from build123d import *

# Parameters (mm, degrees)
CROQUIS1_R               = 0.5
SALIENTE_EXTRUIR1_DEPTH  = 3
SALIENTE_EXTRUIR2_DEPTH  = 11
SALIENTE_EXTRUIR3_DEPTH  = 5.75
CROQUIS4_R               = 2
CROQUIS4_R_2             = 1
CORTAR_EXTRUIR1_DEPTH    = 4
SALIENTE_EXTRUIR5_START  = 4
CROQUIS6_R               = 2
CROQUIS6_R_2             = 1
SALIENTE_EXTRUIR5_DEPTH  = 4
SALIENTE_EXTRUIR6_DEPTH  = 1.5
CROQUIS9_W               = 44.5
CROQUIS9_H               = 15.5
SALIENTE_EXTRUIR7_DEPTH  = 1
CROQUIS11_W              = 10.5
CROQUIS11_H              = 15.5
SALIENTE_EXTRUIR10_DEPTH = 2
CROQUIS7_R               = 2.25
CORTAR_EXTRUIR2_DEPTH    = 2


with BuildPart() as part:
    # Croquis1 → Saliente-Extruir1 (new body)
    with BuildSketch(Plane(origin=(0, 0, 0), x_dir=(1, 0, 0), z_dir=(0, 1, 0))):
        Polygon((-6, -0.75), (-6, -5.5), (4, -5.5), (13.5, -5.5), (13.5, 26.5), (13.5, 39), (4, 39), (4, 26.5), (-6, 26.5), (-6, 21.75), (4, 21.75), (6, 21.75), (6, 11.25), (6, -0.75), align=None)
        with Locations(Location((0, -3.125, 0), (0, 0, 270))):
            Circle(CROQUIS1_R, mode=Mode.SUBTRACT)
        with Locations(Location((0, 24.125, 0), (0, 0, 270))):
            Circle(CROQUIS1_R, mode=Mode.SUBTRACT)
    extrude(amount=SALIENTE_EXTRUIR1_DEPTH)

    # Croquis2 → Saliente-Extruir2 (add)
    with BuildSketch(Plane(origin=(0, 3, 0), x_dir=(1, 0, 0), z_dir=(0, 1, 0))):
        Polygon((11.25, -5.5), (13.5, -5.5), (13.5, 26.5), (13.5, 39), (4, 39), (4, 26.5), (4, 21.75), (6, 21.75), (6, 12.75), (7.25, 12.75), (7.25, 33), (11.25, 33), align=None)
    extrude(amount=SALIENTE_EXTRUIR2_DEPTH)

    # Croquis3 → Saliente-Extruir3 (add)
    with BuildSketch(Plane(origin=(0, 3, 0), x_dir=(1, 0, 0), z_dir=(0, 1, 0))):
        Polygon((11.25, -5.5), (11.25, 33), (7.25, 33), (7.25, 12.75), (6, 12.75), (6, -5.5), align=None)
    extrude(amount=SALIENTE_EXTRUIR3_DEPTH)

    # Croquis4 → Cortar-Extruir1 (cut)
    with BuildSketch(Plane(origin=(0, 0, -39), x_dir=(-1, 0, 0), z_dir=(0, 0, -1))):
        with Locations((-9.87, 11.055)):
            Circle(CROQUIS4_R)
        with Locations((-9.87, 5.555)):
            Circle(CROQUIS4_R_2)
        with Locations((-9.87, 2.055)):
            Circle(CROQUIS4_R_2)
    extrude(amount=-CORTAR_EXTRUIR1_DEPTH, mode=Mode.SUBTRACT)

    # Croquis6 → Saliente-Extruir5 (add)
    with BuildSketch(Plane(origin=(0, 0, -35), x_dir=(-1, 0, 0), z_dir=(0, 0, -1)).offset(SALIENTE_EXTRUIR5_START)):
        with Locations((-9.87, 11.055)):
            Circle(CROQUIS6_R)
        with Locations((-9.87, 5.555)):
            Circle(CROQUIS6_R_2)
        with Locations((-9.87, 2.055)):
            Circle(CROQUIS6_R_2)
    extrude(amount=-SALIENTE_EXTRUIR5_DEPTH)

    # Croquis8 → Saliente-Extruir6 (add)
    with BuildSketch(Plane(origin=(0, 14, 0), x_dir=(1, 0, 0), z_dir=(0, 1, 0))):
        Polygon((4, 39), (4, 21.75), (6, 21.75), (6, 12.75), (7.25, 12.75), (7.25, 33), (11.25, 33), (11.25, -5.5), (13.5, -5.5), (13.5, 39), align=None)
    extrude(amount=SALIENTE_EXTRUIR6_DEPTH)

    # Croquis9 → Saliente-Extruir7 (add)
    with BuildSketch(Plane(origin=(13.5, 0, 0), x_dir=(0, 0, -1), z_dir=(1, 0, 0))):
        with Locations((16.75, 7.75)):
            Rectangle(CROQUIS9_W, CROQUIS9_H)
    extrude(amount=SALIENTE_EXTRUIR7_DEPTH)

    # Croquis11 → Saliente-Extruir10 (add)
    with BuildSketch(Plane(origin=(0, 0, -39), x_dir=(-1, 0, 0), z_dir=(0, 0, -1))):
        with Locations((-9.25, 7.75)):
            Rectangle(CROQUIS11_W, CROQUIS11_H)
    extrude(amount=SALIENTE_EXTRUIR10_DEPTH)

    # Croquis7 → Cortar-Extruir2 (cut)
    with BuildSketch(Plane(origin=(0, 0, -41), x_dir=(-1, 0, 0), z_dir=(0, 0, -1))):
        with Locations((-9.87, 11.055)):
            Circle(CROQUIS7_R)
    extrude(amount=-CORTAR_EXTRUIR2_DEPTH, mode=Mode.SUBTRACT)


solid = part.part
Build history of the part. All positions in model axes, mm. A direction names the side the tool comes from. Round coordinates to 2 decimals unless told otherwise and drop trailing zeros. Order: outer loops, then holes, each group sorted by start corner. A loop starts at its lowest first (then second) coordinate and runs counter-clockwise, first axis right, second up. Notation, with made-up numbers: M 22.5,37.25 L 63.5,37.25 A28 ccw 63.5,70.25 Z; hole C 89,76.5 d8. An arc over 180 degrees is marked long. Use CSV: the item, a comma, the result in double quotes. Start each with the question number.
(1) Mould opens along X. For faces 4 (the face through (11.25, 12, -14)), 5 (the face through (14.5, 8, -17)), 6 (the face through (4.4, 4.3, -21.75)) say: +X half, -X half, draft (parallel to the pull), parting line (faces both ways), or undercut.
(2) Cut at D-D on z = -36. List the corners of the cut face in (x, y), then the cut area to 3 significant figures.
(3) Cut at A-A on x = 1.5. List the corners of the cut face in (y, z), then the cut area to 3 significant figures.
(4) Cut at B-B on y = 14.5. List the corners of the cut face in (x, z).
(5) Tool access for faces 1 (the face through (9, 12, -33)), 2 (the face through (10, 11, -39)), 3 (the face through (7, 12, -12.75)): list every direction of +Z, -Z, +X, -X, +Y, -Y with a clear straight run to the whole face (end or side of a thin tool).
(6) Drill centre lines: probe 1 along X at (y, z) = (10.75, -13.5); probe 2 along X at (y, z) = (11.5, -22.5); probe 3 along X at (y, z) = (10, 4). Where is each one in solid material? Low to high.
(7) Cut at C-C on x = 9.87. List the corners of the cut face in (y, z) (3 decimals).
(8) Flat gauge pins, fed straight in: P1, Ø5, axis at x = 2, z = 4, coming from the +Y side; P2, Ø2, axis at y = 6.5, z = -9.5, coming from the -X side; P3, Ø2, axis at x = 10.5, y = 11.5, coming from the -Z side; P4, Ø4.5, axis at x = 10, y = 11, coming from the +Z side. Where does each tip first touch, or does it go through?
Findings:
1,face 4,"undercut"
1,face 5,"+X half"
1,face 6,"draft"
2,outline,"M 4,0 L 14.5,0 L 14.5,15.5 L 4,15.5 Z"
2,area,"163 mm^2"
3,outline,"M 0,-26.5 L 3,-26.5 L 3,-21.75 L 0,-21.75 Z; M 0,0.75 L 3,0.75 L 3,5.5 L 0,5.5 Z"
3,area,"28.5 mm^2"
4,outline,"M 4,-41 L 14.5,-41 L 14.5,5.5 L 11.25,5.5 L 11.25,-33 L 7.25,-33 L 7.25,-12.75 L 6,-12.75 L 6,-21.75 L 4,-21.75 Z"
5,face 1,"+Z, +Y"
5,face 2,"-Z"
5,face 3,"+Z, -X, +Y"
6,probe 1,"x = 6 to 7.25, 11.25 to 14.5"
6,probe 2,"x = 4 to 7.25, 11.25 to 14.5"
6,probe 3,"x = 11.25 to 14.5"
7,outline,"M 0,-41 L 8.805,-41 L 8.805,-39 L 13.305,-39 L 13.305,-41 L 15.5,-41 L 15.5,-33 L 8.75,-33 L 8.75,5.5 L 0,5.5 Z"
8,P1,"stops at y = 3"
8,P2,"stops at x = 6"
8,P3,"stops at z = -39"
8,P4,"stops at z = 5.5"
